The listing builds one solid part. Answer for the finished solid, in the listing's coordinates (mm). Give positions to 0.01 mm unless a question says otherwise; leave off trailing zeros. Write each loop counter-clockwise with the first axis right and the second up, starting at its lowest first coordinate (ties: lowest second). Pieces come first, ordered by that corner, then holes. Notation, with made-up numbers: M 15,48.5 L 38,48.5 A17 ccw 38,72.5 Z; hole C 16.25,33.5 d11. An arc over 180 degrees is marked long. Answer as a JSON object with one key per item and string values.
```python
from build123d import *

# Parameters (mm, degrees)
F1_DEPTH = 0.64516


with BuildPart() as f1:
    # F0 (on Front) → F1 (new body)
    with BuildSketch(Plane.XZ):
        with BuildLine():
            ThreePointArc((0, 1.27), (0.371974, 0.371974), (1.27, 0))
            Line((1.27, 0), (119.38, 0))
            ThreePointArc((119.38, 0), (120.278026, 0.371974), (120.65, 1.27))
            Line((120.65, 1.27), (120.65, 8.255))
            ThreePointArc((120.65, 8.255), (121.021974, 9.153026), (121.92, 9.525))
            Line((121.92, 9.525), (150.495, 9.525))
            ThreePointArc((150.495, 9.525), (156.332166, 11.942834), (158.75, 17.78))
            Line((158.75, 17.78), (158.75, 36.195))
            ThreePointArc((158.75, 36.195), (156.332166, 42.032166), (150.495, 44.45))
            Line((150.495, 44.45), (142.54871, 44.45))
            ThreePointArc((142.54871, 44.45), (135.497057, 44.123014), (128.505923, 43.144861))
            Line((128.505923, 43.144861), (1.035954, 19.244241))
            ThreePointArc((1.035954, 19.244241), (0.292723, 18.807061), (0, 17.995994))
            Line((0, 17.995994), (0, 1.27))
        make_face()
        with BuildLine():
            ThreePointArc((144.234807, 24.13), (133.35, 28.575), (144.234807, 33.02))
            Line((144.234807, 33.02), (144.234807, 24.13))
        make_face(mode=Mode.SUBTRACT)
    extrude(amount=F1_DEPTH)


solid = f1.part
```
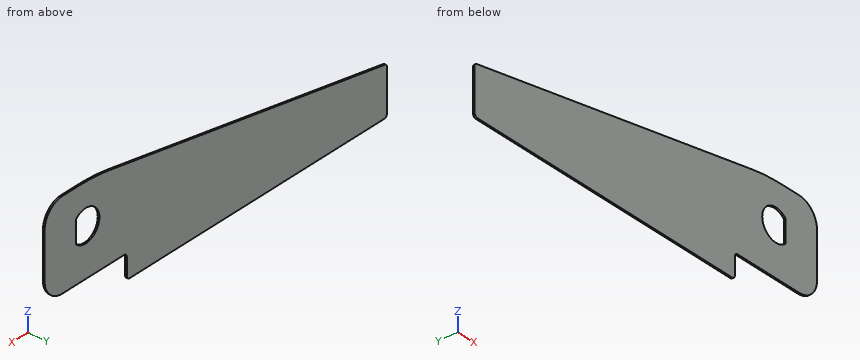
1. A cutting plane is placed at C-C, the plane z = 29.5. Give the vertices of the cut face in (x, y), plus the area to 3 significant figures.
Verdict:
{"outline": "M 55.73,-0.65 L 133.42,-0.65 L 133.42,0 L 55.73,0 Z; M 144.23,-0.65 L 158.75,-0.65 L 158.75,0 L 144.23,0 Z", "area": "59.5 mm2"}
2. Consider line 1 along Z through (x, y) = (139.7, -0.5) (3 decimals); line 2 along X through (y, z) = (-0.3, 13.5); line 3 along Z through (x, y) = (79, -0.6). Determine where each line is inside the solid, lowest interval first.
Verdict:
{"line 1": "z = 9.525 to 22.225, 34.925 to 44.397", "line 2": "x = 0 to 157.55", "line 3": "z = 0 to 33.86"}
3. A flat-ended cylindrical pin translates along its axis: pin 1 (11.5 mm diameter, centred on x = 139.7, z = 28.575, fed in from +Y). Find the tip coordinate at first contact, or state that the pin passes through.
Verdict:
{"pin 1": "stops at y = 0"}
4. A cutting plane is placed at D-D, the plane z = 3.5. Give the vertices of the cut face in (x, y).
Verdict:
{"outline": "M 0,-0.65 L 120.65,-0.65 L 120.65,0 L 0,0 Z"}
5. A cutting plane is placed at B-B, the plane x = 139.7. Give the vertices of the cut face in (y, z) (3 decimals), plus the area to 3 significant figures.
Verdict:
{"outline": "M -0.645,9.525 L 0,9.525 L 0,22.225 L -0.645,22.225 Z; M -0.645,34.925 L 0,34.925 L 0,44.397 L -0.645,44.397 Z", "area": "14.3 mm2"}
6. A cutting plane is placed at A-A, the plane y = -0.5. Give the vertices of the cut face in (x, z) (3 decimals).
Verdict:
{"outline": "M 0,1.27 A1.27 ccw 1.27,0 L 119.38,0 A1.27 ccw 120.65,1.27 L 120.65,8.255 A1.27 cw 121.92,9.525 L 150.495,9.525 A8.255 ccw 158.75,17.78 L 158.75,36.195 A8.255 ccw 150.495,44.45 L 142.549,44.45 A76.2 ccw 128.506,43.145 L 1.036,19.244 A1.27 ccw 0,17.996 Z; hole M 144.235,24.13 L 144.235,33.02 A6.35 ccw long Z"}
